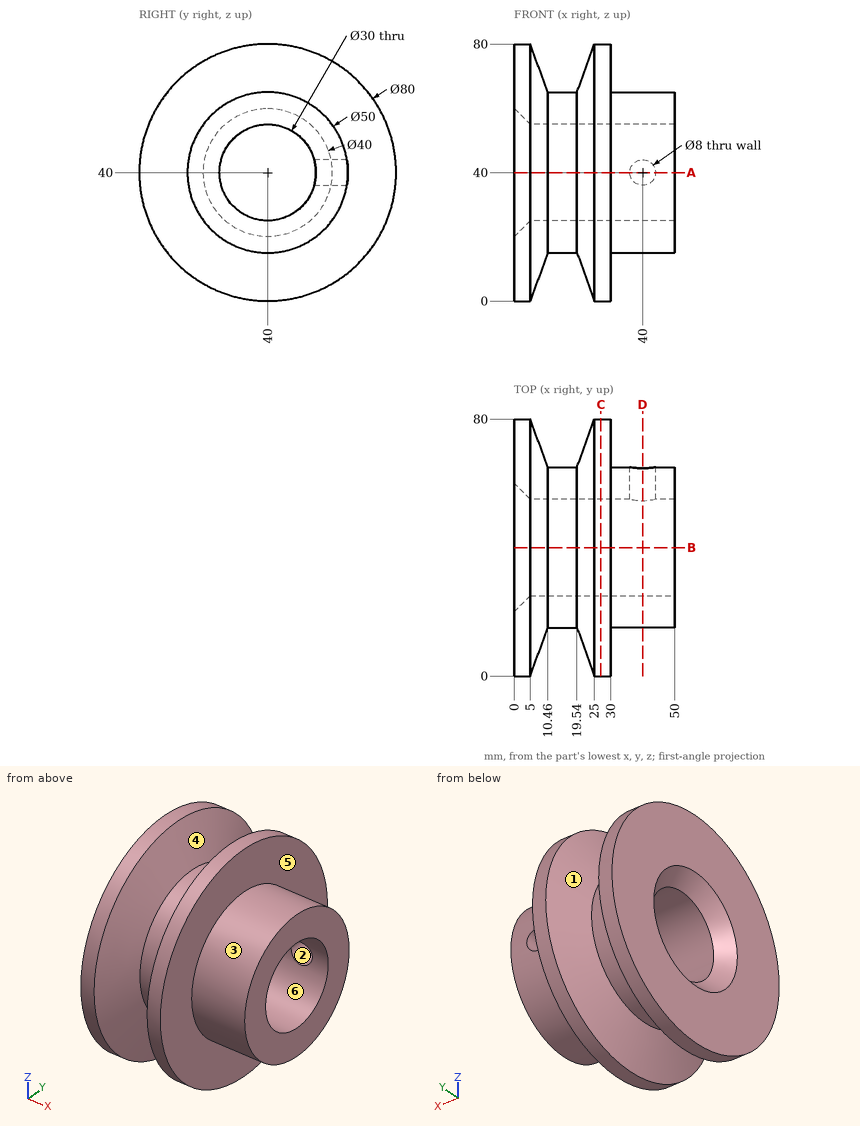
Answer from the drawing. Dimensions are ordinates in mm from the lowest x, y and z of the part. A direction names the side the tool comes from. Coordinates: 2 decimals unless noted, no trailing zeros. Write each loop counter-clockwise with the first axis right and the second up, starting at its lowest first coordinate (ties: lowest second). Pieces come first, ordered by that corner, then holes. Notation, with made-up numbers: (86, -9.5) - (133, -9.5) arc R22 ccw to (133, 11.5) - close; hole circle Ø7 at (47, -37.5). An arc over 180 degrees is marked (long way). Return JSON: item names as keys, results as strings.
1. The part is cut by section D-D on x = 40. Determine the outline of the cut face in (y, z).
Final values:
{"outline": "(54.46, 36) arc R15 cw (long way) to (54.46, 44) - (64.68, 44) arc R25 ccw (long way) to (64.68, 36) - close"}
2. The part is cut by section A-A on z = 40. Determine the outline of the cut face in (x, y).
Final values:
{"outline": "(0, 0) - (5, 0) - (10.46, 15) - (19.54, 15) - (25, 0) - (30, 0) - (30, 15) - (50, 15) - (50, 25) - (5, 25) - (0, 20) - close; (0, 60) - (5, 55) - (36, 55) - (36, 65) - (30, 65) - (30, 80) - (25, 80) - (19.54, 65) - (10.46, 65) - (5, 80) - (0, 80) - close; (44, 55) - (50, 55) - (50, 65) - (44, 65) - close"}
3. For a pull along Y with two mould halves and no side action, classify the marked faces 4, 5 and 6 as +Y half, -Y half, draft (parallel to the pull), parting line (faces both ways), or undercut.
Final values:
{"face 4": "parting line", "face 5": "draft", "face 6": "undercut"}
4. Which of the six approach directions +Z, -Z, +X, -X, +Y, -Y give full straight-line access (tool end or side, diameter ignored) to the marked faces 1, 2 and 3?
Final values:
{"face 1": "none", "face 2": "+Y", "face 3": "+X"}
5. The part is cut by section B-B on y = 40. Determine the outline of the cut face in (x, z), then the cut area to 3 significant figures.
Final values:
{"outline": "(0, 0) - (5, 0) - (10.46, 15) - (19.54, 15) - (25, 0) - (30, 0) - (30, 15) - (50, 15) - (50, 25) - (5, 25) - (0, 20) - close; (0, 60) - (5, 55) - (50, 55) - (50, 65) - (30, 65) - (30, 80) - (25, 80) - (19.54, 65) - (10.46, 65) - (5, 80) - (0, 80) - close", "area": "1,440 mm^2"}
6. Consider line 1 along Y through (x, z) = (16, 40.5) (1 decimal); line 2 along Z through (x, y) = (29, 40). Determine where each line is inside the solid, lowest interval first.
Final values:
{"line 1": "15 to 25, 55 to 65", "line 2": "0 to 25, 55 to 80"}
7. Each of these flat-tipped pins is pushed along its axis until it touches: pin 1 Ø3 at (x, y) = (27, 39.5) entering from -Z; pin 2 Ø13 at (x, z) = (40, 40) entering from +Y; pin 3 Ø1.5 at (x, y) = (31.5, 22.5) entering from -Z. Where does it stop, or does it pass through?
Final values:
{"pin 1": "z = 0", "pin 2": "y = 65", "pin 3": "z = 21.44"}
8. The part is cut by section C-C on x = 27. Determine the outline of the cut face in (y, z), then the cut area to 3 significant figures.
Final values:
{"outline": "circle Ø80 at (40, 40); hole circle Ø30 at (40, 40)", "area": "4,320 mm^2"}
